from build123d import *

# Parameters (mm, degrees)
SKETCH1_W            = 629.90984
SKETCH1_H            = 147.69846
BOSS_EXTRUDE1_DEPTH  = 3.175
SKETCH3_W            = 254
SKETCH3_H            = 3.175
BOSS_EXTRUDE2_DEPTH  = 6.35
SKETCH4_W            = 3.175
SKETCH4_H            = 188.732840052
CUT_EXTRUDE1_DEPTH   = 3.175
SKETCH6_W            = 3.175
SKETCH6_H            = 110.773845
BOSS_EXTRUDE4_DEPTH  = 3.175
SKETCH8_W            = 629.90984
SKETCH8_H            = 18.04416
BOSS_EXTRUDE5_DEPTH  = 3.175
SKETCH10_W           = 38.1
SKETCH10_H           = 36.08832
CUT_EXTRUDE3_DEPTH   = 652.56536379
SKETCH12_W           = 38.1
SKETCH12_H           = 18.04416
BOSS_EXTRUDE7_DEPTH  = 3.175
SKETCH17_W           = 38.1
SKETCH17_H           = 18.04416
CUT_EXTRUDE5_DEPTH   = 652.56536379
SKETCH18_W           = 38.1
SKETCH18_H           = 18.450049938
CUT_EXTRUDE6_DEPTH   = 652.56536379
SKETCH24_W           = 5.08
SKETCH24_H           = 12.7
CUT_EXTRUDE11_DEPTH  = 652.56536379
M4_CLEARANCE_HOLE3_D = 4.8


with BuildPart() as part:
    # Sketch1 → Boss-Extrude1 (new body)
    with BuildSketch(Plane(origin=(0, 0, 0), x_dir=(1, 0, 0), z_dir=(0, 1, 0))):
        with Locations((314.95492, 73.84923)):
            Rectangle(SKETCH1_W, SKETCH1_H)
    extrude(amount=BOSS_EXTRUDE1_DEPTH)

    # Sketch3 → Boss-Extrude2 (add)
    with BuildSketch(Plane(origin=(0, 0, -147.69846), x_dir=(-1, 0, 0), z_dir=(0, 0, -1))):
        with Locations((-473.22613, 1.5875)):
            Rectangle(SKETCH3_W, SKETCH3_H)
        with Locations((-156.68371, 1.5875)):
            Rectangle(SKETCH3_W, SKETCH3_H)
    extrude(amount=BOSS_EXTRUDE2_DEPTH)

    # Sketch4 → Cut-Extrude1 (cut)
    with BuildSketch(Plane(origin=(0, 3.175, 0), x_dir=(1, 0, 0), z_dir=(0, 1, 0))):
        with Locations((314.95492, 147.69846)):
            Rectangle(SKETCH4_W, SKETCH4_H)
    extrude(amount=-CUT_EXTRUDE1_DEPTH, mode=Mode.SUBTRACT)

    # Sketch6 → Boss-Extrude4 (add)
    with BuildSketch(Plane(origin=(0, 3.175, 0), x_dir=(1, 0, 0), z_dir=(0, 1, 0))):
        with Locations((631.49734, 92.3115375)):
            Rectangle(SKETCH6_W, SKETCH6_H)
        with Locations((-1.5875, 92.3115375)):
            Rectangle(SKETCH6_W, SKETCH6_H)
    extrude(amount=-BOSS_EXTRUDE4_DEPTH)

    # Sketch8 → Boss-Extrude5 (add, through all)
    with BuildSketch(Plane(origin=(0, 3.175, 0), x_dir=(1, 0, 0), z_dir=(0, 1, 0))):
        with Locations((314.95492, -9.02208)):
            Rectangle(SKETCH8_W, SKETCH8_H)
    extrude(amount=-BOSS_EXTRUDE5_DEPTH)

    # Sketch10 → Cut-Extrude3 (cut, through all)
    with BuildSketch(Plane(origin=(0, 3.175, 0), x_dir=(1, 0, 0), z_dir=(0, 1, 0))):
        with Locations((579.10984, -18.04416)):
            Rectangle(SKETCH10_W, SKETCH10_H)
        with Locations((50.8, -18.04416)):
            Rectangle(SKETCH10_W, SKETCH10_H)
    extrude(amount=-CUT_EXTRUDE3_DEPTH, mode=Mode.SUBTRACT)

    # Sketch12 → Boss-Extrude7 (add, through all)
    with BuildSketch(Plane(origin=(0, 3.175, 0), x_dir=(1, 0, 0), z_dir=(0, 1, 0))):
        with Locations((50.8, -9.02208)):
            Rectangle(SKETCH12_W, SKETCH12_H)
        with Locations((579.10984, -9.02208)):
            Rectangle(SKETCH12_W, SKETCH12_H)
    extrude(amount=-BOSS_EXTRUDE7_DEPTH)

    # Sketch17 → Cut-Extrude5 (cut, through all)
    with BuildSketch(Plane(origin=(0, 3.175, 0), x_dir=(1, 0, 0), z_dir=(0, 1, 0))):
        with Locations((262.56742, -9.02208)):
            Rectangle(SKETCH17_W, SKETCH17_H)
        with Locations((367.34242, -9.02208)):
            Rectangle(SKETCH17_W, SKETCH17_H)
    extrude(amount=-CUT_EXTRUDE5_DEPTH, mode=Mode.SUBTRACT)

    # Sketch18 → Cut-Extrude6 (cut, through all)
    with BuildSketch(Plane(origin=(0, 3.175, 0), x_dir=(1, 0, 0), z_dir=(0, 1, 0))):
        with Locations((73.1774, -8.819135031)):
            Rectangle(SKETCH18_W, SKETCH18_H)
        with Locations((548.657320006, -8.819135031)):
            Rectangle(SKETCH18_W, SKETCH18_H)
    extrude(amount=-CUT_EXTRUDE6_DEPTH, mode=Mode.SUBTRACT)

    # Sketch24 → Cut-Extrude11 (cut, through all)
    with BuildSketch(Plane(origin=(0, 3.175, 0), x_dir=(1, 0, 0), z_dir=(0, 1, 0))):
        with Locations((2.54, -11.69416)):
            Rectangle(SKETCH24_W, SKETCH24_H)
        with Locations((627.36984, -11.69416)):
            Rectangle(SKETCH24_W, SKETCH24_H)
    extrude(amount=-CUT_EXTRUDE11_DEPTH, mode=Mode.SUBTRACT)

    # M4 Clearance Hole3 (through all)
    with Locations(Plane(origin=(0, 3.175, 0), x_dir=(1, 0, 0), z_dir=(0, 1, 0))):
        with Locations((44.409412743, -5.996840051), (156.68371, -5.996840051), (194.108475752, -5.996840051), (294.859886505, -5.996840051), (335.049953495, -5.996840051), (435.801364248, -5.996840051), (473.22613, -5.996840051), (510.650895752, -5.996840051), (585.500427257, -5.996840051)):
            Hole(M4_CLEARANCE_HOLE3_D / 2)


solid = part.part
Geometry: final body of the model. Coordinates: model frame, mm. Coordinates: 2 decimals unless noted, no trailing zeros. Order: outer loops, then holes, each group sorted by start corner. A loop starts at its lowest first (then second) coordinate and runs counter-clockwise, first axis right, second up.
(1) Section query B-B (y = 0.75). State how many separate pieces and enclosed holes the cut face has, plus the area to 3 significant figures.
(2) Material intervals for probe 1 along X at (y, z) = (1.4, -63) (3 decimals); probe 2 along X at (y, z) = (2.1, 10.5); probe 3 along Z at (x, y) = (75.5, 1.45), sorted ascending.
(3) First-contact query: pin 1 (1.6 mm diameter, centred on y = 1.5, z = 11.5, fed in from -X); pin 2 (4 mm diameter, centred on x = 473.23, z = 6, fed in from +Y); pin 3 (1 mm diameter, centred on y = 2, z = 10, fed in from +X); pin 4 (1.5 mm diameter, centred on y = 1, z = -30, fed in from +X). Flat tips, straight axial feed; report the tip coordinate or a pass-through.
(4) Section query A-A (x = 71). Return the cut outline in (y, z) (3 decimals).
Solution:
1. separate pieces: 1
1. enclosed holes: 9
1. area: 105,000 mm2
2. probe 1: x = -3.175 to 313.367, 316.542 to 633.085
2. probe 2: x = 5.08 to 54.13, 92.23 to 243.52, 281.62 to 348.29, 386.39 to 529.61, 567.71 to 624.83
2. probe 3: z = -154.05 to -0.41
3. pin 1: stops at x = 5.08
3. pin 2: passes through
3. pin 3: stops at x = 624.83
3. pin 4: stops at x = 629.91
4. outline: (0, -154.048) - (3.175, -154.048) - (3.175, -0.406) - (0, -0.406) - close
